Could you check a few things on this model? Use its own coordinates, in mm. Give positions to 0.01 mm unless a question says otherwise; leave off trailing zeros. Order: outer loops, then holes, each group sorted by start corner. A loop starts at its lowest first (then second) coordinate and runs counter-clockwise, first axis right, second up. Notation, with made-up numbers: (-39, 70) - (-28, 70) arc R24 cw to (-28, 94) - close; hole circle Ø9 at (48.5, 65). An arc over 180 degrees is marked (long way). Put each result on its own line as item: value.
from build123d import *

# Parameters (mm, degrees)
SKETCH_1_R      = 1.8
EXTRUDE_1_DEPTH = 3


with BuildPart() as part:
    # 草图1 → 凸台-拉伸1 (new body)
    with BuildSketch(Plane(origin=(0, 0, 0), x_dir=(1, 0, 0), z_dir=(0, 1, 0))):
        with BuildLine():
            Line((-90, 10), (-90, 0))
            Line((-90, 0), (-86.8, 0))
            Line((-86.8, 0), (-86.8, 10))
            Line((-86.8, 10), (86.8, 10))
            Line((86.8, 10), (86.8, 0))
            Line((86.8, 0), (90, 0))
            Line((90, 0), (90, 10))
            Line((90, 10), (105, 10))
            ThreePointArc((105, 10), (108.535533906, 8.535533906), (110, 5))
            Line((110, 5), (110, -5))
            ThreePointArc((110, -5), (108.535533906, -8.535533906), (105, -10))
            Line((105, -10), (-105, -10))
            ThreePointArc((-105, -10), (-108.535533906, -8.535533906), (-110, -5))
            Line((-110, -5), (-110, 5))
            ThreePointArc((-110, 5), (-108.535533906, 8.535533906), (-105, 10))
            Line((-105, 10), (-90, 10))
        make_face()
        with Locations(Location((-100, 0, 0), (0, 0, 270))):
            Circle(SKETCH_1_R, mode=Mode.SUBTRACT)
        with Locations(Location((100, 0, 0), (0, 0, 270))):
            Circle(SKETCH_1_R, mode=Mode.SUBTRACT)
    extrude(amount=EXTRUDE_1_DEPTH)


solid = part.part
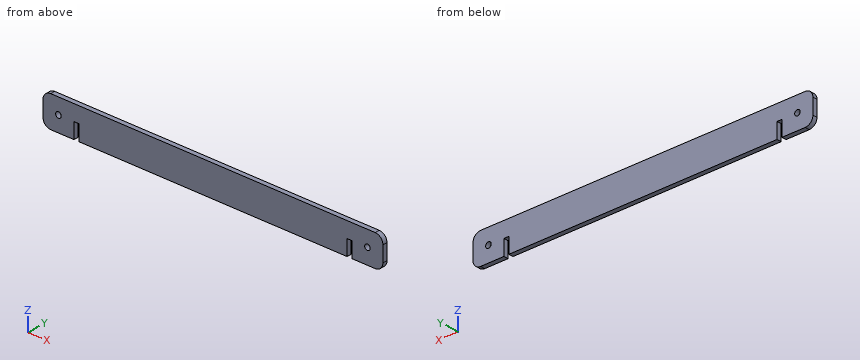
1) Suppose I cut it at A-A, the plane x = 100. List the corners of the cut face in (y, z) for me.
Filled in:
outline: (0, -10) - (3, -10) - (3, -1.8) - (0, -1.8) - close; (0, 1.8) - (3, 1.8) - (3, 10) - (0, 10) - close
2) I'm going to push a flat-ended pin straight in: pin 1 (2 mm diameter, centred on x = 100, z = 0, fed in from +Y). Where does the tip first touch, or does it pass through?
Filled in:
pin 1: passes through
3) Suppose I cut it at B-B, the plane y = 0.75. List the corners of the cut face in (x, z) for me.
Filled in:
outline: (-110, -5) arc R5 ccw to (-105, -10) - (-90, -10) - (-90, 0) - (-86.8, 0) - (-86.8, -10) - (86.8, -10) - (86.8, 0) - (90, 0) - (90, -10) - (105, -10) arc R5 ccw to (110, -5) - (110, 5) arc R5 ccw to (105, 10) - (-105, 10) arc R5 ccw to (-110, 5) - close; hole circle Ø3.6 at (-100, 0); hole circle Ø3.6 at (100, 0)
4) If I drill on line 1 (X direction, y = 2.3, z = -0.25); line 2 (Z direction, x = -100, y = 1.4); line 3 (X direction, y = 0.2, z = -4), over which ranges is the centre line in solid material (lowest first)? Write a range as [from, to].
Filled in:
line 1: x = [-110, -101.78], [-98.22, -90], [-86.8, 86.8], [90, 98.22], [101.78, 110]
line 2: z = [-10, -1.8], [1.8, 10]
line 3: x = [-110, -90], [-86.8, 86.8], [90, 110]
